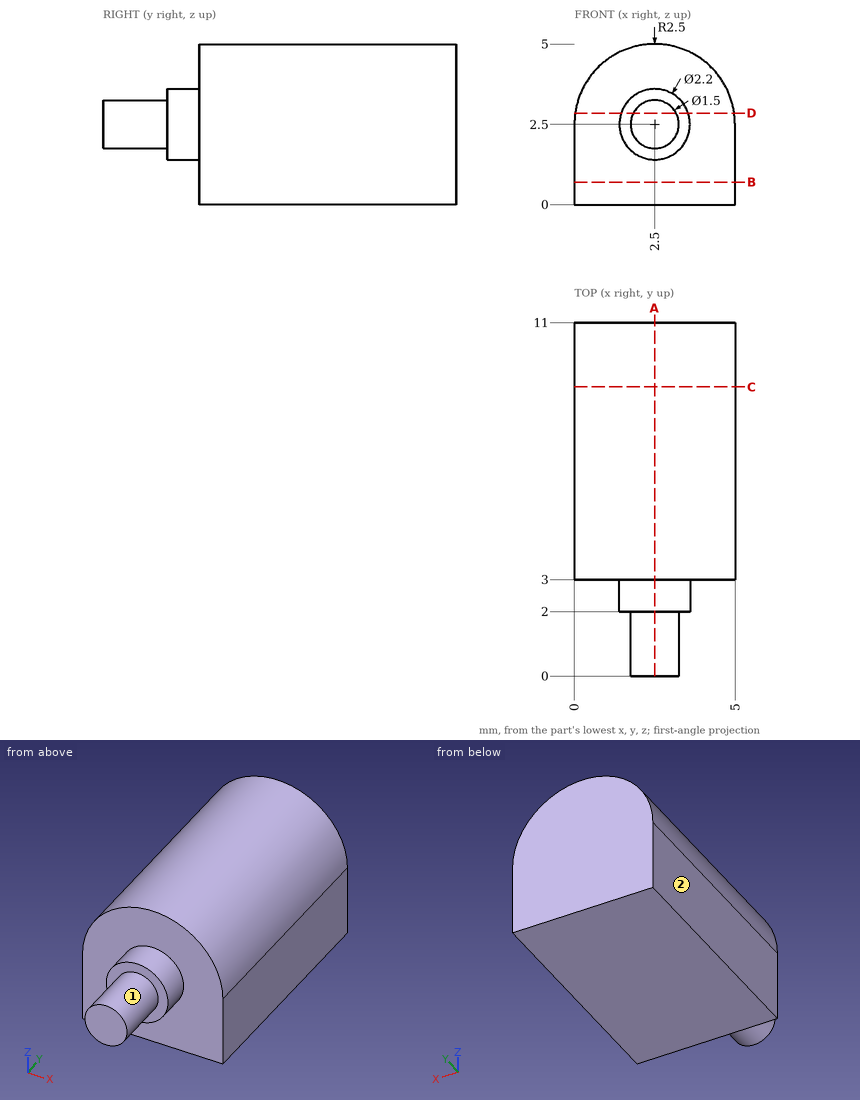
Drawing for the job (mm, zero at the part's lowest x, y, z). A direction names the side the tool comes from. Coordinates: 2 decimals unless noted, no trailing zeros. Loops run counter-clockwise (first coordinate to the right, second up) from the corner with the lowest first, then second, coordinate; pieces in that order, holes last. Notation, with made-up numbers: (36, 15.25) - (63, 15.25) arc R28 cw to (63, 50.25) - close; hole circle Ø2 at (53.25, 29). An arc over 180 degrees is marked (long way). Return JSON: item names as keys, results as strings.
1. Band-saw the part on C-C (y = 9). Give the cut face in (x, z).
Result:
{"outline": "(0, 0) - (5, 0) - (5, 2.5) arc R2.5 ccw to (0, 2.5) - close"}
2. Probe L1, parallel to Y at x = 3.85, z = 2.85; L2, parallel to Z at x = 4.75, y = 8.5; L3, parallel to Z at x = 3.95, y = 4.5. List the from-to ranges inside material, lowest first. Write a range as from..to.
Result:
{"L1": "y = 3..11", "L2": "z = 0..3.59", "L3": "z = 0..4.54"}
3. Drop a flat-ended pin along its axis: pin 1 (3 mm diameter, centred on y = 7.5, z = 4.5, fed in from +X). Give the stop position or say it passes through.
Result:
{"pin 1": "stops at x = 4.95"}
4. Band-saw the part on B-B (z = 0.7). Give the cut face in (x, y), and give its area (3 significant figures).
Result:
{"outline": "(0, 3) - (5, 3) - (5, 11) - (0, 11) - close", "area": "40.0 mm2"}
5. Band-saw the part on D-D (z = 2.85). Give the cut face in (x, y).
Result:
{"outline": "(0.02, 3) - (1.46, 3) - (1.46, 2) - (1.84, 2) - (1.84, 0) - (3.16, 0) - (3.16, 2) - (3.54, 2) - (3.54, 3) - (4.98, 3) - (4.98, 11) - (0.02, 11) - close"}
6. Band-saw the part on A-A (x = 2.5). Give the cut face in (y, z).
Result:
{"outline": "(0, 1.75) - (2, 1.75) - (2, 1.4) - (3, 1.4) - (3, 0) - (11, 0) - (11, 5) - (3, 5) - (3, 3.6) - (2, 3.6) - (2, 3.25) - (0, 3.25) - close"}
7. 3-axis set-ups, long thin cutter, end or side, ignore diameter. For the marked faces 1 and 2: which of +Z, -Z, +X, -X, +Y, -Y reach the whole face in a straight line?
Result:
{"face 1": "-Y", "face 2": "+Z, -Z, -X, +Y, -Y"}
